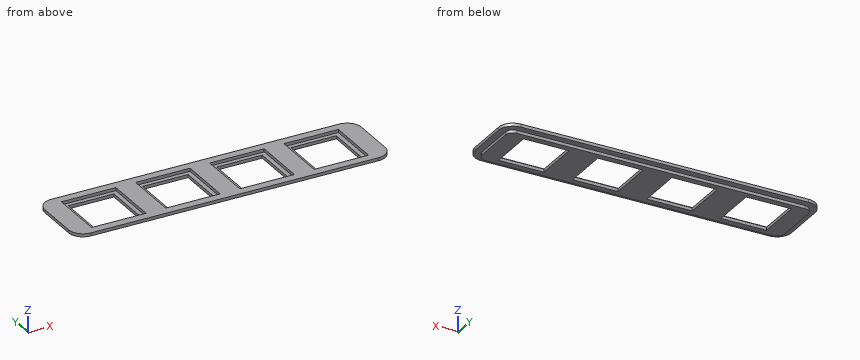
```python
from build123d import *

# Parameters (mm, degrees)
BOSS_EXTRU_1_DEPTH      = 2
BOSS_EXTRU_3_DEPTH      = 2
ESQUISSE7_W             = 36
ESQUISSE7_H             = 36
ENL_V_MAT_EXTRU_4_DEPTH = 2
ESQUISSE8_W             = 30.1
ESQUISSE8_H             = 30.1
ENL_V_MAT_EXTRU_5_DEPTH = 108.195394024


with BuildPart() as part:
    # Esquisse1 → Boss.-Extru.1 (new body)
    with BuildSketch(Plane.XY):
        with BuildLine():
            Line((-95, -23.55), (95, -23.55))
            ThreePointArc((95, -23.55), (101.717514421, -20.767514421), (104.5, -14.05))
            Line((104.5, -14.05), (104.5, 14.05))
            ThreePointArc((104.5, 14.05), (101.717514421, 20.767514421), (95, 23.55))
            Line((95, 23.55), (-95, 23.55))
            ThreePointArc((-95, 23.55), (-101.717514421, 20.767514421), (-104.5, 14.05))
            Line((-104.5, 14.05), (-104.5, -14.05))
            ThreePointArc((-104.5, -14.05), (-101.717514421, -20.767514421), (-95, -23.55))
        make_face()
    extrude(amount=BOSS_EXTRU_1_DEPTH)

    # Esquisse6 → Boss.-Extru.3 (add)
    with BuildSketch(Plane(origin=(0, 0, 0), x_dir=(-1, 0, 0), z_dir=(0, 0, -1))):
        with BuildLine():
            Line((-95, -19.05), (95, -19.05))
            ThreePointArc((95, -19.05), (98.535533906, -17.585533906), (100, -14.05))
            Line((100, -14.05), (100, 14.05))
            ThreePointArc((100, 14.05), (98.535533906, 17.585533906), (95, 19.05))
            Line((95, 19.05), (-95, 19.05))
            ThreePointArc((-95, 19.05), (-98.535533906, 17.585533906), (-100, 14.05))
            Line((-100, 14.05), (-100, -14.05))
            ThreePointArc((-100, -14.05), (-98.535533906, -17.585533906), (-95, -19.05))
        make_face()
    extrude(amount=BOSS_EXTRU_3_DEPTH)

    # Esquisse7 → Enlèv. mat.-Extru.4 (cut)
    with BuildSketch(Plane.XY.offset(2)):
        with Locations((-73.5, 0)):
            Rectangle(ESQUISSE7_W, ESQUISSE7_H)
        with Locations((-24.5, 0)):
            Rectangle(ESQUISSE7_W, ESQUISSE7_H)
        with Locations((24.5, 0)):
            Rectangle(ESQUISSE7_W, ESQUISSE7_H)
        with Locations((73.5, 0)):
            Rectangle(ESQUISSE7_W, ESQUISSE7_H)
    extrude(amount=-ENL_V_MAT_EXTRU_4_DEPTH, mode=Mode.SUBTRACT)

    # Esquisse8 → Enlèv. mat.-Extru.5 (cut, through all)
    with BuildSketch(Plane(origin=(0, 0, -2), x_dir=(-1, 0, 0), z_dir=(0, 0, -1))):
        with Locations((-73.5, 0)):
            Rectangle(ESQUISSE8_W, ESQUISSE8_H)
        with Locations((-24.5, 0)):
            Rectangle(ESQUISSE8_W, ESQUISSE8_H)
        with Locations((24.5, 0)):
            Rectangle(ESQUISSE8_W, ESQUISSE8_H)
        with Locations((73.5, 0)):
            Rectangle(ESQUISSE8_W, ESQUISSE8_H)
    extrude(amount=-ENL_V_MAT_EXTRU_5_DEPTH, mode=Mode.SUBTRACT)


solid = part.part
```
CAD build for the part. Positions are in the model's coordinates, mm. Round coordinates to 2 decimals unless told otherwise and drop trailing zeros. Write each loop counter-clockwise with the first axis right and the second up, starting at its lowest first coordinate (ties: lowest second). Pieces come first, ordered by that corner, then holes. Notation, with made-up numbers: (30.5, 35) - (74.5, 35) arc R11 cw to (74.5, 54) - close; hole circle Ø3 at (75, 74.5). An arc over 180 degrees is marked (long way). Write item = value, one per line. Start each with the question number.
Q1. Band-saw the part on B-B (x = 21). Give the cut face in (y, z).
Q2. Band-saw the part on C-C (y = -3.5). Count the separate pieces of the cut face and the enclosed holes in it, then the cut area to 3 significant figures.
Q3. Probe L1, parallel to X at y = 4, z = 1.6; L2, parallel to X at y = -9.5, z = -0.8; L3, parallel to Y at x = -74.5, z = 0.25. List the from-to ranges inside material, lowest first. Write a range as from..to.
Q4. Band-saw the part on A-A (z = -0.9). Give the cut face in (x, y), then the cut area to 3 significant figures.
Q5. Drop flat-ended pins along their axis: pin 1 (11 mm diameter, centred on x = -78.5, y = -1.5, fed in from +Z); pin 2 (8 mm diameter, centred on x = 59, y = -13.5, fed in from +Z); pin 3 (2 mm diameter, centred on y = -5.5, z = -1.5, fed in from -X); pin 4 (2 mm diameter, centred on x = -72, z = -1.5, fed in from +Y). Give the stop position or say it passes through.
Answers below:
q1.outline = (-23.55, 0) - (-19.05, 0) - (-19.05, -2) - (-15.05, -2) - (-15.05, 0) - (-18, 0) - (-18, 2) - (-23.55, 2) - close; (15.05, -2) - (19.05, -2) - (19.05, 0) - (23.55, 0) - (23.55, 2) - (18, 2) - (18, 0) - (15.05, 0) - close
q2.separate_pieces = 5
q2.enclosed_holes = 0
q2.area = 289 mm2
q3.L1 = -104.5..-91.5, -55.5..-42.5, -6.5..6.5, 42.5..55.5, 91.5..104.5
q3.L2 = -100..-88.55, -58.45..-39.55, -9.45..9.45, 39.55..58.45, 88.55..100
q3.L3 = -23.55..-18, 18..23.55
q4.outline = (-100, -14.05) arc R5 ccw to (-95, -19.05) - (95, -19.05) arc R5 ccw to (100, -14.05) - (100, 14.05) arc R5 ccw to (95, 19.05) - (-95, 19.05) arc R5 ccw to (-100, 14.05) - close; hole (-88.55, -15.05) - (-58.45, -15.05) - (-58.45, 15.05) - (-88.55, 15.05) - close; hole (-39.55, -15.05) - (-9.45, -15.05) - (-9.45, 15.05) - (-39.55, 15.05) - close; hole (9.45, -15.05) - (39.55, -15.05) - (39.55, 15.05) - (9.45, 15.05) - close; hole (58.45, -15.05) - (88.55, -15.05) - (88.55, 15.05) - (58.45, 15.05) - close
q4.area = 3,970 mm2
q5.pin_1 = through
q5.pin_2 = 2
q5.pin_3 = -100
q5.pin_4 = 19.05
